```python
from build123d import *

# Parameters (mm, degrees)
F0_W      = 33
F0_H      = 38
F0_W_2    = 27
F0_H_2    = 32
F1_DEPTH  = 6
F2_DEPTH  = 2
F4_D      = 2.2
F4_DEPTH  = 5
F4_TIP    = 0.6609466809
F5_W      = 10
F5_H      = 6
F6_DEPTH  = 6
F7_W      = 10
F7_H      = 6
F8_DEPTH  = 6
F10_D     = 2.2
F10_DEPTH = 5
F10_TIP   = 0.6609466809
F11_W     = 20
F11_H     = 3
F12_DEPTH = 3
F13_W     = 20
F13_H     = 3
F14_DEPTH = 2
F15_W     = 11
F15_H     = 15
F16_DEPTH = 2
F3_R      = 7.5
F17_DEPTH = 2.001


with BuildPart() as f1:
    # F0 (on Top) → F1 (new body)
    with BuildSketch(Plane.XY):
        Rectangle(F0_W, F0_H)
        Rectangle(F0_W_2, F0_H_2, mode=Mode.SUBTRACT)
    extrude(amount=F1_DEPTH)

    # F0 (on Top) → F2 (join)
    with BuildSketch(Plane.XY):
        Rectangle(F0_W_2, F0_H_2)
    extrude(amount=F2_DEPTH)

    # F4
    with Locations(Plane(origin=(0, 0, 0), x_dir=(1, 0, 0), z_dir=(0, 0, -1))):
        with Locations((-10.75, 0.5), (-10.75, -12.5), (10.75, -12.5), (10.75, 0.5)):
            Hole(F4_D / 2, depth=F4_DEPTH)
            with Locations((0, 0, -(F4_DEPTH + F4_TIP / 2))):  # 118° drill point
                Cone(0, F4_D / 2, F4_TIP, mode=Mode.SUBTRACT)

    # F5 (on face) → F6 (join)
    with BuildSketch(Plane.YZ.offset(16.5)):
        with Locations((0, 3)):
            Rectangle(F5_W, F5_H)
    extrude(amount=F6_DEPTH)

    # F7 (on face) → F8 (join)
    with BuildSketch(Plane(origin=(-16.5, 0, 0), x_dir=(0, -1, 0), z_dir=(-1, 0, 0))):
        with Locations((0, 3)):
            Rectangle(F7_W, F7_H)
    extrude(amount=F8_DEPTH)

    # F10
    with Locations(Plane(origin=(0, 0, 0), x_dir=(1, 0, 0), z_dir=(0, 0, -1))):
        with Locations((20.625, 0), (-20.625, 0)):
            Hole(F10_D / 2, depth=F10_DEPTH)
            with Locations((0, 0, -(F10_DEPTH + F10_TIP / 2))):  # 118° drill point
                Cone(0, F10_D / 2, F10_TIP, mode=Mode.SUBTRACT)

    # F11 (on face) → F12 (cut, through all)
    with BuildSketch(Plane.XZ.offset(19)):
        with Locations((0, 4.5)):
            Rectangle(F11_W, F11_H)
    extrude(amount=-F12_DEPTH, mode=Mode.SUBTRACT)

    # F13 (on face) → F14 (join)
    with BuildSketch(Plane.XZ.offset(19)):
        with Locations((0, 1.5)):
            Rectangle(F13_W, F13_H)
    extrude(amount=F14_DEPTH)

    # F15 (on face) → F16 (cut)
    with BuildSketch(Plane.XY.offset(3)):
        with Locations((0, 6)):
            Rectangle(F15_W, F15_H)
    extrude(amount=-F16_DEPTH, mode=Mode.SUBTRACT)

    # F3 (on face) → F17 (cut, through all)
    with BuildSketch(Plane(origin=(0, 0, 0), x_dir=(1, 0, 0), z_dir=(0, 0, -1))):
        with Locations((0, 0.5)):
            Circle(F3_R)
    extrude(amount=-F17_DEPTH, mode=Mode.SUBTRACT)


solid = f1.part
```
Source: CAD feature listing. Evaluate the final solid. Frame: model axes, mm. A direction names the side the tool comes from. Coordinates: 2 decimals unless noted, no trailing zeros. Write each loop counter-clockwise with the first axis right and the second up, starting at its lowest first coordinate (ties: lowest second). Pieces come first, ordered by that corner, then holes. Notation, with made-up numbers: M 30,41.5 L 58,41.5 A13 ccw 58,56.5 Z; hole C -6.75,54.25 d8. An arc over 180 degrees is marked long. Answer as a JSON object with one key per item and string values.
1. Cut plane B-B on x = 0. Output: boundary loops of the cut face in (y, z).
Evaluation:
{"outline": "M -21,0 L -8,0 L -8,2 L -16,2 L -16,3 L -21,3 Z; M 7,0 L 19,0 L 19,6 L 16,6 L 16,2 L 13.5,2 L 13.5,1 L 7,1 Z"}
2. Access query for faces 5 (the flat face through (19, 5, 3)), 6 (the flat face through (-16.5, -12, 3)), 7 (the flat face through (-0.2, -16, 2.6)). Directions: +Z, -Z, +X, -X, +Y, -Y. A direction counts if a zero-diameter tool reaches every point of the face in a straight line with its end or side. Return the directions, or none.
Evaluation:
{"face 5": "+Z, -Z, +X, +Y", "face 6": "+Z, -Z, -X, -Y", "face 7": "+Z"}
3. Cut plane C-C on x = 10.75. Output: boundary loops of the cut face in (y, z), plus the area to 3 significant figures.
Evaluation:
{"outline": "M -19,0 L -1.6,0 L -1.6,2 L -16,2 L -16,6 L -19,6 Z; M 0.6,0 L 11.4,0 L 11.4,2 L 0.6,2 Z; M 13.6,0 L 19,0 L 19,6 L 16,6 L 16,2 L 13.6,2 Z", "area": "91.2 mm^2"}
4. Ray query, L1, parallel to X at y = 12.5, z = 1.25; L2, parallel to Y at x = -10.75, z = 1; L3, parallel to X at y = 12.5, z = 0.9. Return the intervals inside material, ascending.
Evaluation:
{"L1": "-16.5 to -11.85, -9.65 to -5.5, 5.5 to 9.65, 11.85 to 16.5", "L2": "-19 to -1.6, 0.6 to 11.4, 13.6 to 19", "L3": "-16.5 to -11.85, -9.65 to 9.65, 11.85 to 16.5"}
5. Draft query along Y for faces 1 (the flat face through (13.5, 0, 4)), 2 (the flat face through (10, -18, 4)), 3 (the flat face through (-19, 5, 3)), 4 (the cylindrical face through (-11.766, -0.079, 1.014)). Return one class per face: released by +Y, released by -Y, zero draft, split by the parting line, or undercut.
Evaluation:
{"face 1": "undercut", "face 2": "zero draft", "face 3": "released by +Y", "face 4": "undercut"}
6. Cut plane A-A on z = 4.2. Output: boundary loops of the cut face in (x, y) (3 decimals), plus the area to 3 significant figures.
Evaluation:
{"outline": "M -22.5,-5 L -16.5,-5 L -16.5,-19 L -10,-19 L -10,-16 L -13.5,-16 L -13.5,16 L 13.5,16 L 13.5,-16 L 10,-16 L 10,-19 L 16.5,-19 L 16.5,-5 L 22.5,-5 L 22.5,5 L 16.5,5 L 16.5,19 L -16.5,19 L -16.5,5 L -22.5,5 Z; hole C -20.625,0 d2.2; hole C 20.625,0 d2.2", "area": "442 mm^2"}
7. Contact query for flat-ended pins moving along their axis: P1, Ø3, axis at y = 7.5, z = 1, coming from the -X side; P2, Ø1, axis at y = 14, z = 2.5, coming from the +X side; P3, Ø2.5, axis at x = -1.5, y = 7.5, coming from the +Z side. Output: stop coordinate, or through.
Evaluation:
{"P1": "x = -16.5", "P2": "x = 16.5", "P3": "z = 1"}
8. Cut plane D-D on y = 2.5. Output: boundary loops of the cut face in (x, z), plus the area to 3 significant figures.
Evaluation:
{"outline": "M -22.5,0 L -6.87,0 L -6.87,2 L -13.5,2 L -13.5,6 L -22.5,6 Z; M 6.87,0 L 22.5,0 L 22.5,6 L 13.5,6 L 13.5,2 L 6.87,2 Z", "area": "135 mm^2"}
